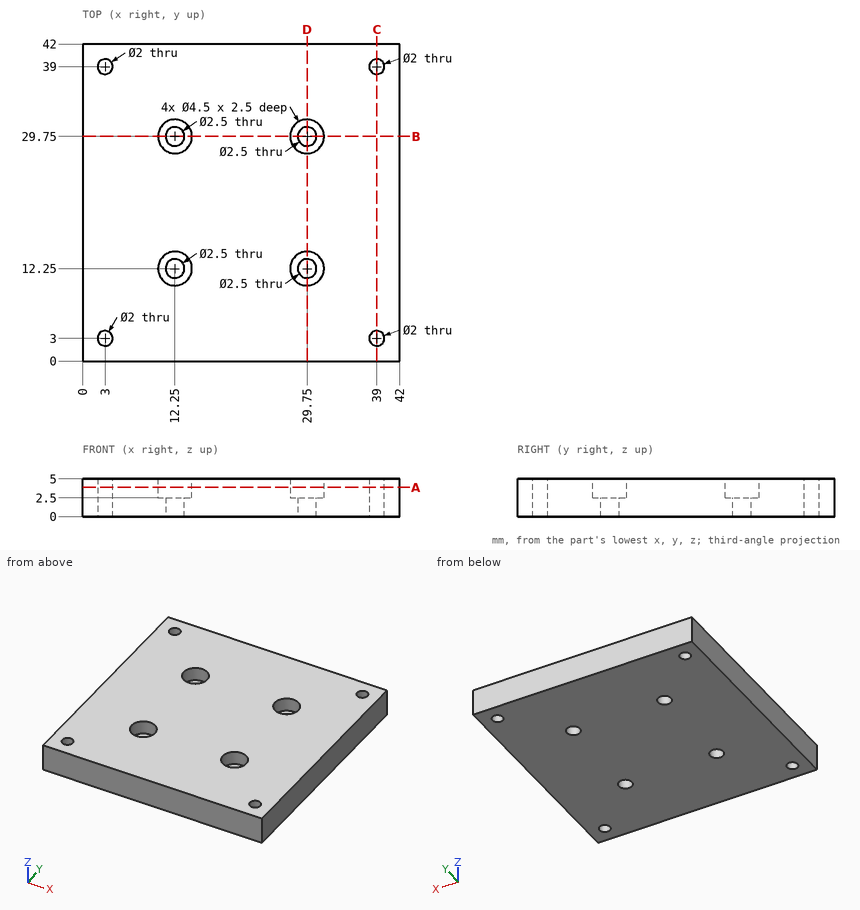
Geometry: see drawing. Coordinates: mm, zero at the bounding-box minimum. Give positions to 0.01 mm unless a question says otherwise; leave off trailing zeros. Order: outer loops, then holes, each group sorted by start corner. A loop starts at its lowest first (then second) coordinate and runs counter-clockwise, first axis right, second up. Notation, with made-up numbers: (10, 87.25) - (46, 87.25) arc R16 cw to (46, 109.25) - close; hole circle Ø3 at (52, 71). An arc over 180 degrees is marked (long way). One line per item, written item: value.
1. Cut plane B-B, the plane y = 29.75. Output: boundary loops of the cut face in (x, z), and give its area (3 significant figures).
Determined:
outline: (0, 0) - (11, 0) - (11, 2.5) - (10, 2.5) - (10, 5) - (0, 5) - close; (13.5, 0) - (28.5, 0) - (28.5, 2.5) - (27.5, 2.5) - (27.5, 5) - (14.5, 5) - (14.5, 2.5) - (13.5, 2.5) - close; (31, 0) - (42, 0) - (42, 5) - (32, 5) - (32, 2.5) - (31, 2.5) - close
area: 175 mm2
2. Pin query (flat end, axial travel): pin 1 Ø4 at (x, y) = (16, 8.5) entering from -Z; pin 2 Ø3.5 at (x, y) = (29.75, 12.25) entering from +Z. Return the tip coordinate at first contact, or that it passes through.
Determined:
pin 1: z = 0
pin 2: z = 2.5
3. Line query: probe 1 along Y at (x, z) = (29.75, 3.65); probe 2 along Y at (x, z) = (39, 2.25). Output: solid intervals per line, ascending.
Determined:
probe 1: 0 to 10, 14.5 to 27.5, 32 to 42
probe 2: 0 to 2, 4 to 38, 40 to 42
4. Cut plane A-A, the plane z = 3.9. Give the number of separate pieces and of enclosed holes in the cut face, and give its area (3 significant figures).
Determined:
separate pieces: 1
enclosed holes: 8
area: 1,690 mm2
5. Cut plane C-C, the plane x = 39. Output: boundary loops of the cut face in (y, z).
Determined:
outline: (0, 0) - (2, 0) - (2, 5) - (0, 5) - close; (4, 0) - (38, 0) - (38, 5) - (4, 5) - close; (40, 0) - (42, 0) - (42, 5) - (40, 5) - close
